Check sheet for the drawn part. Datum: minimum x, y, z corner. Units: mm. Round coordinates to 2 decimals unless told otherwise and drop trailing zeros. Write each loop counter-clockwise with the first axis right and the second up, starting at its lowest first coordinate (ties: lowest second). Pieces come first, ordered by that corner, then holes. Notation, with made-up numbers: (9.25, 32) -> (63.25, 32) arc R25 ccw to (63.25, 47) -> close; hole circle Ø4 at (-5.75, 40). An arc over 180 degrees is marked (long way). Use CSV: the item, a comma, the result in double quotes.
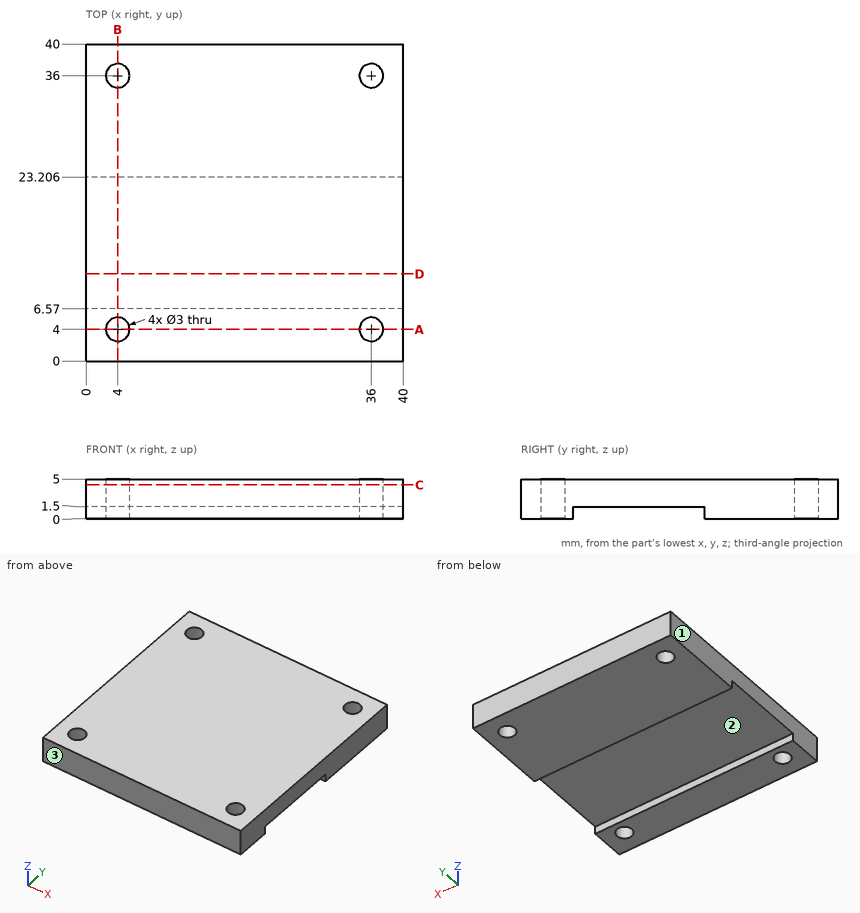
Q1. Section check C-C (z = 4.25). Record the cut outline in (x, y), plus the area to 3 significant figures.
Filled in:
outline,"(0, 0) -> (40, 0) -> (40, 40) -> (0, 40) -> close; hole circle Ø3 at (4, 4); hole circle Ø3 at (4, 36); hole circle Ø3 at (36, 4); hole circle Ø3 at (36, 36)"
area,"1,570 mm²"
Q2. Mould release check, pull along Y, two halves, no side actions. Record for the marked faces 1, 2 and 3: released by +Y, released by -Y, zero draft, split by the parting line, or undercut.
Filled in:
face 1,"zero draft"
face 2,"undercut"
face 3,"released by -Y"
Q3. Section check B-B (x = 4). Record the cut outline in (y, z).
Filled in:
outline,"(0, 0) -> (2.5, 0) -> (2.5, 5) -> (0, 5) -> close; (5.5, 0) -> (6.57, 0) -> (6.57, 1.5) -> (23.21, 1.5) -> (23.21, 0) -> (34.5, 0) -> (34.5, 5) -> (5.5, 5) -> close; (37.5, 0) -> (40, 0) -> (40, 5) -> (37.5, 5) -> close"
Q4. Section check A-A (y = 4). Record the cut outline in (x, z).
Filled in:
outline,"(0, 0) -> (2.5, 0) -> (2.5, 5) -> (0, 5) -> close; (5.5, 0) -> (34.5, 0) -> (34.5, 5) -> (5.5, 5) -> close; (37.5, 0) -> (40, 0) -> (40, 5) -> (37.5, 5) -> close"
Q5. Material ranges on L1, parallel to Y at x = 36, z = 4.85; L2, parallel to Y at x = 4, z = 1; L3, parallel to Y at x = 27, z = 0.45, recorded low to high.
Filled in:
L1,"0 to 2.5, 5.5 to 34.5, 37.5 to 40"
L2,"0 to 2.5, 5.5 to 6.57, 23.21 to 34.5, 37.5 to 40"
L3,"0 to 6.57, 23.21 to 40"
Q6. Go/stop test with flat-tipped pins: P1, Ø5, axis at x = 21, y = 12.5, coming from the -Z side; P2, Ø3.5, axis at x = 4, y = 4, coming from the +Z side. Record where each tip stops, or that it passes through.
Filled in:
P1,"z = 1.5"
P2,"z = 5"
Q7. Section check D-D (y = 11). Record the cut outline in (x, z), plus the area to 3 significant figures.
Filled in:
outline,"(0, 1.5) -> (40, 1.5) -> (40, 5) -> (0, 5) -> close"
area,"140 mm²"
